Source: CAD feature listing. Evaluate the final solid. Frame: model axes, mm. Face numbers are marked on the shaded views. A direction names the side the tool comes from. Give positions to 0.01 mm unless a question says otherwise; leave off trailing zeros. Order: outer loops, then holes, each group sorted by start corner. A loop starts at its lowest first (then second) coordinate and runs counter-clockwise, first axis right, second up. Notation, with made-up numbers: M -3,-30 L 25,-30 A19 ccw 25,-24 Z; hole C 39.5,-21 d2. An arc over 180 degrees is marked long. Use CSV: the item, a comma, the result in double quotes. Start each with the question number.
1. Section query D-D, the plane y = -6. Return the cut outline in (x, z), plus the area to 3 significant figures.
2. Line query: line 1 along Z through (x, y) = (-8, -6); line 2 along Z through (x, y) = (-15, 13.5); line 3 along X through (y, z) = (12, 57.5). Output: solid intervals per line, ascending. Write a range as [from, to].
3. Section query C-C, the plane z = 51. Return the cut outline in (x, y), plus the area to 3 significant figures.
4. Pin query (flat end, axial travel): P1, Ø1.5, axis at y = -12, z = 56, coming from the -X side; P2, Ø6, axis at x = -10.5, y = -9, coming from the +Z side; P3, Ø1.5, axis at x = -4.5, y = -1.5, coming from the +Z side. Return the tip coordinate at first contact, or that it passes through.
5. Reachability of the marked faces 1 and 2 from +Z, -Z, +X, -X, +Y, -Y: full face, straight path, thin tool, end or side. Return the list, or none.
6. Section query A-A, the plane y = 0. Return the cut outline in (x, z).
from build123d import *

# Parameters (mm, degrees)
SKETCH1_W           = 35
SKETCH1_H           = 35
BOSS_EXTRUDE1_DEPTH = 30.8
SKETCH2_R           = 16
BOSS_EXTRUDE2_DEPTH = 33
SKETCH4_R           = 9.5
BOSS_EXTRUDE4_DEPTH = 2
SKETCH3_R           = 3
BOSS_EXTRUDE3_DEPTH = 15.94


with BuildPart() as part:
    # Sketch1 → Boss-Extrude1 (new body)
    with BuildSketch(Plane.XY):
        Rectangle(SKETCH1_W, SKETCH1_H)
    extrude(amount=BOSS_EXTRUDE1_DEPTH)

    # Sketch2 → Boss-Extrude2 (add)
    with BuildSketch(Plane.XY.offset(30.8)):
        Circle(SKETCH2_R)
    extrude(amount=BOSS_EXTRUDE2_DEPTH)

    # Sketch4 → Boss-Extrude4 (add)
    with BuildSketch(Plane.XY.offset(63.8)):
        Circle(SKETCH4_R)
    extrude(amount=BOSS_EXTRUDE4_DEPTH)

    # Sketch3 → Boss-Extrude3 (add)
    with BuildSketch(Plane.XY.offset(65.8)):
        Circle(SKETCH3_R)
    extrude(amount=BOSS_EXTRUDE3_DEPTH)


solid = part.part
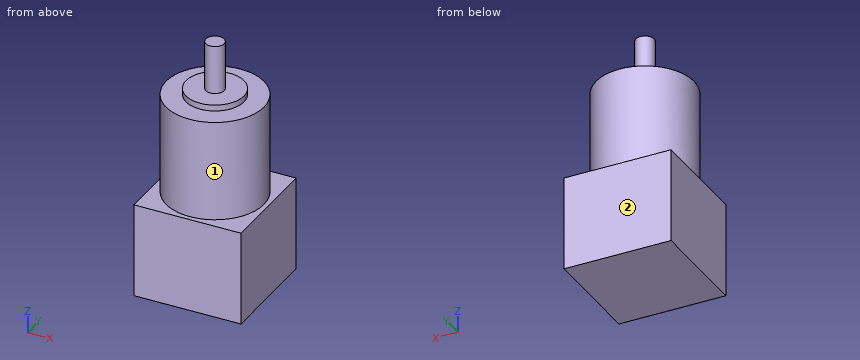
Result set:
1,outline,"M -17.5,0 L 17.5,0 L 17.5,30.8 L 14.83,30.8 L 14.83,63.8 L 7.37,63.8 L 7.37,65.8 L -7.37,65.8 L -7.37,63.8 L -14.83,63.8 L -14.83,30.8 L -17.5,30.8 Z"
1,area,"2,090 mm2"
2,line 1,"[0, 63.8]"
2,line 2,"[0, 30.8]"
2,line 3,"[-10.58, 10.58]"
3,outline,"C 0,0 d32"
3,area,"804 mm2"
4,P1,"x = -11.38"
4,P2,"z = 63.8"
4,P3,"z = 65.8"
5,face 1,"+Z"
5,face 2,"+Z, -Z, +X, -X, +Y"
6,outline,"M -17.5,0 L 17.5,0 L 17.5,30.8 L 16,30.8 L 16,63.8 L 9.5,63.8 L 9.5,65.8 L 3,65.8 L 3,81.74 L -3,81.74 L -3,65.8 L -9.5,65.8 L -9.5,63.8 L -16,63.8 L -16,30.8 L -17.5,30.8 Z"
